from build123d import *

# Parameters (mm, degrees)
GRUNDPLATTE_KREUZ_DEPTH         = 2
MITTELBOHRUNG_DEPTH             = 12.489125293
MITTELBOHRUNG_DEPTH_BACK        = 12.489125293
SKIZZE11_R                      = 1.25
SKIZZE12_R                      = 3.25
AUFSATZ_LINEAR_AUSTRAGEN2_DEPTH = 2
FASE1_SIZE                      = 0.25
SKIZZE13_R                      = 2.35
SCHNITT_LINEAR_AUSTRAGEN1_DEPTH = 4


with BuildPart() as part:
    # Skizze4 → Grundplatte Kreuz (new body)
    with BuildSketch(Plane(origin=(0, 0, 0), x_dir=(1, 0, 0), z_dir=(0, 1, 0))):
        Polygon((-8, -2), (-8, 2), (-3.5, 2), (-3.5, 8), (3.5, 8), (3.5, 2), (8, 2), (8, -2), (3.5, -2), (3.5, -8), (-3.5, -8), (-3.5, -2), align=None)
    extrude(amount=GRUNDPLATTE_KREUZ_DEPTH)

    # Skizze11 → Mittelbohrung (cut, two sides: drawn at the far end of the back side and taken through both)
    with BuildSketch(Plane(origin=(0, 0, 0), x_dir=(1, 0, 0), z_dir=(0, 1, 0)).offset(-MITTELBOHRUNG_DEPTH_BACK)):
        with Locations(Location((0, 0, 0), (0, 0, 270))):
            Circle(SKIZZE11_R)
    extrude(amount=MITTELBOHRUNG_DEPTH + MITTELBOHRUNG_DEPTH_BACK, mode=Mode.SUBTRACT)

    # Skizze12 → Aufsatz-Linear austragen2 (add)
    with BuildSketch(Plane.XZ):
        with Locations(Location((0, 0, 0), (0, 0, 90))):
            Circle(SKIZZE12_R)
    extrude(amount=AUFSATZ_LINEAR_AUSTRAGEN2_DEPTH)

    # Fase1
    fase1_edges = [part.edges().sort_by_distance(p)[0] for p in [
        (0, -2, -3.25),
    ]]
    chamfer(fase1_edges, length=FASE1_SIZE)

    # Skizze13 → Schnitt-Linear austragen1 (cut)
    with BuildSketch(Plane.XZ.offset(2)):
        with Locations(Location((0, 0, 0), (0, 0, 270))):
            Circle(SKIZZE13_R)
    extrude(amount=-SCHNITT_LINEAR_AUSTRAGEN1_DEPTH, mode=Mode.SUBTRACT)


solid = part.part
Design review of the part built by this model. Coordinates are the model's own, in mm. A direction names the side the tool comes from. Round coordinates to 2 decimals unless told otherwise and drop trailing zeros. Loops run counter-clockwise (first coordinate to the right, second up) from the corner with the lowest first, then second, coordinate; pieces in that order, holes last. Notation, with made-up numbers: (46.5, -24.5) - (54.5, -24.5) arc R21 cw to (54.5, -18.5) - close; hole circle Ø5 at (10.5, -13.5). An arc over 180 degrees is marked (long way). One line per item, written item: value. Start each with the question number.
1) Draft analysis for pull direction X (two halves, no side actions). For faces 1 (the flat face through (-6, 1, -2)), 2 (the flat face through (3.5, 1, -5)), 3 (the cylindrical face through (0.71, -0.03, -2.24)), state which applies: +X half, -X half, draft (parallel to the pull), parting line (faces both ways), or undercut.
2) Insertion check: pin 1 Ø2 at (x, y) = (6.5, 1.5) entering from -Z; pin 2 Ø5 at (x, z) = (1.5, 1.5) entering from -Y; pin 3 Ø1 at (x, y) = (-6.5, 1.5) entering from +Z; pin 4 Ø2 at (y, z) = (1, -4.5) entering from +X. Each pin has a flat end and moves straight along its axis. Give the tip position at first contact, or say it passes through.
3) Consider section A-A on y = 1.15. Give the boundary of the cut face in (x, z).
4) Consider section D-D on z = 5. Give the boundary of the cut face in (x, y).
5) To check wall thickness, follow L1, parallel to X at y = 0.6, z = 0; L2, parallel to X at y = -0.05, z = 0; L3, parallel to Y at x = 2.5, z = 5.25. State the ranges of each line that lie inside material, in increasing order. Write a range as from..to.
6) Consider section C-C on z = 0. Give the boundary of the cut face in (x, y).
7) Consider section B-B on x = 0. Give the boundary of the cut face in (y, z).
8) For faces 4 (the flat face through (-3.5, 1, -5)), 5 (the cylindrical face through (1.978, -0.863, -2.579)), 6 (the flat face through (3.5, 1, 5)), 7 (the flat face through (-6, 1, 2)), 8 (the flat face through (6, 1, -2)), list the 3-axis set-ups (+Z, -Z, +X, -X, +Y, -Y) from which the entire face can be reached by the end or side of a thin tool; tool diameter is ignored.
Reported:
1. face 1: draft
1. face 2: +X half
1. face 3: undercut
2. pin 1: stops at z = -2
2. pin 2: stops at y = -2
2. pin 3: stops at z = 2
2. pin 4: stops at x = 3.5
3. outline: (-8, -2) - (-3.5, -2) - (-3.5, -8) - (3.5, -8) - (3.5, -2) - (8, -2) - (8, 2) - (3.5, 2) - (3.5, 8) - (-3.5, 8) - (-3.5, 2) - (-8, 2) - close; hole circle Ø4.7 at (0, 0)
4. outline: (-3.5, 0) - (3.5, 0) - (3.5, 2) - (-3.5, 2) - close
5. L1: x = -8..-2.35, 2.35..8
5. L2: x = -3.25..-2.35, 2.35..3.25
5. L3: y = 0..2
6. outline: (-8, 0) - (-3.25, 0) - (-3.25, -1.75) - (-3, -2) - (-2.35, -2) - (-2.35, 2) - (-8, 2) - close; (2.35, -2) - (3, -2) - (3.25, -1.75) - (3.25, 0) - (8, 0) - (8, 2) - (2.35, 2) - close
7. outline: (-2, -3) - (-1.75, -3.25) - (0, -3.25) - (0, -8) - (2, -8) - (2, -2.35) - (-2, -2.35) - close; (-2, 2.35) - (2, 2.35) - (2, 8) - (0, 8) - (0, 3.25) - (-1.75, 3.25) - (-2, 3) - close
8. face 4: -Z, -X, +Y, -Y
8. face 5: -Y
8. face 6: +Z, +X, +Y, -Y
8. face 7: +Z, -X, +Y, -Y
8. face 8: -Z, +X, +Y, -Y
